```python
from build123d import *

# Parameters (mm, degrees)
F0_R     = 150
F1_DEPTH = 50
F2_R     = 20
F3_R     = 108.901018
F4_DEPTH = 25
F5_R     = 10
F6_DEPTH = 150


with BuildPart() as f1:
    # F0 (on Top) → F1 (new body, symmetric)
    with BuildSketch(Plane.XY):
        Circle(F0_R)
    extrude(amount=F1_DEPTH, both=True)

    # F2
    f2_edges = [f1.edges().sort_by_distance(p)[0] for p in [
        (-150, 0, 50),
        (-150, 0, -50),
    ]]
    fillet(f2_edges, radius=F2_R)

    # F3 (on face) → F4 (cut)
    with BuildSketch(Plane.XY.offset(50)):
        Circle(F3_R)
    extrude(amount=-F4_DEPTH, mode=Mode.SUBTRACT)

    # F5 (on face) → F6 (cut)
    with BuildSketch(Plane.XY.offset(25)):
        Circle(F5_R)
    extrude(amount=-F6_DEPTH, mode=Mode.SUBTRACT)


solid = f1.part
```
Work out the finished part from the listing and answer in its coordinate system (mm). A direction names the side the tool comes from. Coordinates: 2 decimals unless noted, no trailing zeros. Loops run counter-clockwise (first coordinate to the right, second up) from the corner with the lowest first, then second, coordinate; pieces in that order, holes last. Notation, with made-up numbers: (17, -23.5) - (62, -23.5) arc R14 ccw to (62, -8.5) - close; hole circle Ø8 at (79, -33.75). An arc over 180 degrees is marked (long way). Use a Markdown table: item, result.
Item 1: Find section A-A, the plane x = 0. Determine the outline of the cut face in (y, z).
Evaluation:
| item | result |
|---|---|
| outline | (-150, -30) arc R20 ccw to (-130, -50) - (-10, -50) - (-10, 25) - (-108.9, 25) - (-108.9, 50) - (-130, 50) arc R20 ccw to (-150, 30) - close; (10, -50) - (130, -50) arc R20 ccw to (150, -30) - (150, 30) arc R20 ccw to (130, 50) - (108.9, 50) - (108.9, 25) - (10, 25) - close |
Item 2: The mould has two halves that part along X. Classify faces 1 (the cylindrical face through (-2.17, -9.76, -11.98)), 2 (the cylindrical face through (-19.527, 148.724, 0.42)), 3 (the flat face through (-29.5, -105.3, 50)): +X half, -X half, draft (parallel to the pull), parting line (faces both ways), or undercut.
Evaluation:
| item | result |
|---|---|
| face 1 | undercut |
| face 2 | parting line |
| face 3 | draft |
Item 3: Find section C-C, the plane z = 19.5. Determine the outline of the cut face in (x, y), and give its area (3 significant figures).
Evaluation:
| item | result |
|---|---|
| outline | circle Ø300 at (0, 0); hole circle Ø20 at (0, 0) |
| area | 70,400 mm2 |
Item 4: Given pin 1 Ø6 at (x, z) = (115, 1) entering from +Y; pin 2 Ø2 at (y, z) = (-55, -33) entering from -X; pin 3 Ø10 at (x, y) = (-65.5, 66.5) entering from +Z; pin 4 Ø18 at (x, y) = (0, 0) entering from +Z, each flat-ended and moving along its own axis, determine where each tip first touches the part or whether it passes through.
Evaluation:
| item | result |
|---|---|
| pin 1 | stops at y = 99.78 |
| pin 2 | stops at x = -139.73 |
| pin 3 | stops at z = 25 |
| pin 4 | passes through |
Item 5: Find section D-D, the plane z = 37. Determine the outline of the cut face in (x, y) (3 decimals), and give its area (3 significant figures).
Evaluation:
| item | result |
|---|---|
| outline | circle Ø297.47 at (0, 0); hole circle Ø217.802 at (0, 0) |
| area | 32,200 mm2 |
Item 6: Consider probe 1 along Y at (x, z) = (0, -26); probe 2 along Y at (x, z) = (0, 31); probe 3 along X at (y, z) = (-5.5, -42). Determine where each line is inside the solid, lowest interval first. Write a range as from..to.
Evaluation:
| item | result |
|---|---|
| probe 1 | y = -150..-10, 10..150 |
| probe 2 | y = -149.97..-108.9, 108.9..149.97 |
| probe 3 | x = -145.9..-8.35, 8.35..145.9 |
Item 7: For faces 4 (the flat face through (27, 2, -50)), 5 (the cylindrical face through (50.251, -96.614, 37.675)), determine the directions among +Z, -Z, +X, -X, +Y, -Y from which every point of the face is accessible in a straight line to the end or side of a thin tool.
Evaluation:
| item | result |
|---|---|
| face 4 | -Z, +X, -X, +Y, -Y |
| face 5 | +Z |
